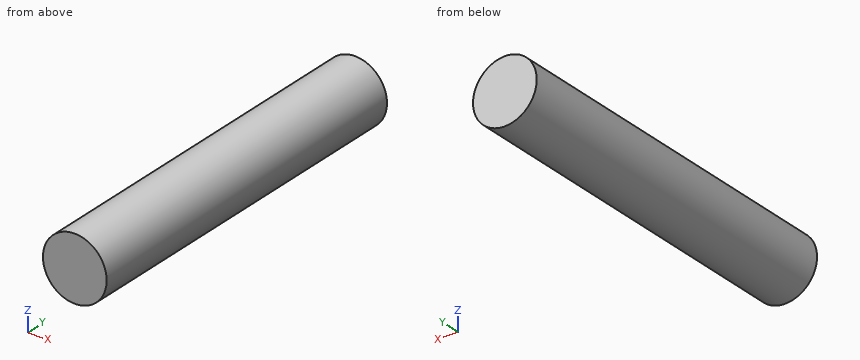
from build123d import *

# Parameters (mm, degrees)
F0_R     = 9.5208183928
F1_DEPTH = 101.6
F3_R     = 11.0662804661
F4_DEPTH = 127


with BuildPart() as f1:
    # F0 (on Front) → F1 (new body)
    with BuildSketch(Plane.XZ):
        Circle(F0_R)
    extrude(amount=F1_DEPTH)


with BuildPart() as f4:
    # F3 (on Front) → F4 (new body)
    with BuildSketch(Plane.XZ):
        Circle(F3_R)
    extrude(amount=F4_DEPTH)


solid = f4.part
Model file for the job. Use its own axes, mm. Give positions to 0.01 mm unless a question says otherwise; leave off trailing zeros. Order: outer loops, then holes, each group sorted by start corner. A loop starts at its lowest first (then second) coordinate and runs counter-clockwise, first axis right, second up. Notation, with made-up numbers: M 55.5,-7 L 102.5,-7 A16 ccw 102.5,19 Z; hole C 8.5,25.5 d2. An arc over 180 degrees is marked long. Put each result on its own line as item: value. Start each with the question number.
(1) Pin check, flat tips, straight feed: pin 1 Ø8 at (x, y) = (-2, -29.5) entering from +Z; pin 2 Ø1 at (x, y) = (-1, -23) entering from -Z (3 decimals); pin 3 Ø1.5 at (x, y) = (-5, -84.5) entering from -Z. Stop position of each tip, or through.
(2) Band-saw the part on C-C on z = 9.75. Give the cut face in (x, y), then the cut area to 3 significant figures.
(3) Drill centre lines: L1, parallel to Z at x = 0.75, y = -48.5; L2, parallel to X at y = -102, z = -0.25; L3, parallel to Z at x = -9.5, y = -31.5. Where is each one in solid material? Low to high. Write a range as [from, to].
(4) Band-saw the part on B-B on x = 9.5. Give the cut face in (y, z), then the cut area to 3 significant figures.
(5) Band-saw the part on A-A on y = -56.5. Give the cut face in (x, z), then the cut area to 3 significant figures.
Results below:
1. pin 1: stops at z = 11.07
1. pin 2: stops at z = -11.055
1. pin 3: stops at z = -10.22
2. outline: M -5.23,-127 L 5.23,-127 L 5.23,0 L -5.23,0 Z
2. area: 1,330 mm2
3. L1: z = [-11.04, 11.04]
3. L2: x = [-11.06, 11.06]
3. L3: z = [-5.68, 5.68]
4. outline: M -127,-5.68 L 0,-5.68 L 0,5.68 L -127,5.68 Z
4. area: 1,440 mm2
5. outline: C 0,0 d22.13
5. area: 385 mm2
